CAD build for the part. Positions are in the model's coordinates, mm. A direction names the side the tool comes from. Give positions to 0.01 mm unless a question says otherwise; leave off trailing zeros. Order: outer loops, then holes, each group sorted by start corner. A loop starts at its lowest first (then second) coordinate and runs counter-clockwise, first axis right, second up.
```python
from build123d import *

# Parameters (mm, degrees)
SKETCH1_R           = 0.5
SKETCH1_R_2         = 1.375
BOSS_EXTRUDE1_DEPTH = 2
SKETCH4_R           = 4.6270037
SKETCH4_R_2         = 2.6270037
BOSS_EXTRUDE3_DEPTH = 6.5
CUT_EXTRUDE3_DEPTH  = 6.5
SKETCH6_R           = 15.875
SKETCH6_R_2         = 3.75
BOSS_EXTRUDE6_DEPTH = 2.54
SKETCH7_R           = 1.778
CUT_EXTRUDE4_DEPTH  = 2.54
CIRPATTERN1_COUNT   = 4
ESQUISSE1_R         = 15.875
ESQUISSE1_R_2       = 1.375
ESQUISSE1_R_3       = 1.778
BOSS_EXTRU_1_DEPTH  = 1.46
ESQUISSE2_R         = 4.625
BOSS_EXTRU_2_DEPTH  = 7.8


with BuildPart() as part:
    # Sketch1 → Boss-Extrude1 (new body)
    with BuildSketch(Plane(origin=(0, 0, 0), x_dir=(1, 0, 0), z_dir=(0, 1, 0))):
        with BuildLine():
            Line((-4, 4), (-2.467435953, 13.402193757))
            ThreePointArc((-2.467435953, 13.402193757), (0, 15.5), (2.467435953, 13.402193757))
            Line((2.467435953, 13.402193757), (4, 4))
            Line((4, 4), (12.448472752, 2.459445505))
            ThreePointArc((12.448472752, 2.459445505), (14.5, 0), (12.448472752, -2.459445505))
            Line((12.448472752, -2.459445505), (4, -4))
            Line((4, -4), (2.467435953, -13.402193757))
            ThreePointArc((2.467435953, -13.402193757), (0, -15.5), (-2.467435953, -13.402193757))
            Line((-2.467435953, -13.402193757), (-4, -4))
            Line((-4, -4), (-12.448472752, -2.459445505))
            ThreePointArc((-12.448472752, -2.459445505), (-14.5, 0), (-12.448472752, 2.459445505))
            Line((-12.448472752, 2.459445505), (-4, 4))
        make_face()
        with Locations((0, 12)):
            Circle(SKETCH1_R, mode=Mode.SUBTRACT)
        with Locations((0, 9.5)):
            Circle(SKETCH1_R, mode=Mode.SUBTRACT)
        with Locations((0, 7.5)):
            Circle(SKETCH1_R, mode=Mode.SUBTRACT)
        with Locations((12, 0)):
            Circle(SKETCH1_R, mode=Mode.SUBTRACT)
        with Locations((9.5, 0)):
            Circle(SKETCH1_R, mode=Mode.SUBTRACT)
        with Locations((7.5, 0)):
            Circle(SKETCH1_R, mode=Mode.SUBTRACT)
        with Locations((0, -12)):
            Circle(SKETCH1_R, mode=Mode.SUBTRACT)
        with Locations((0, -9.5)):
            Circle(SKETCH1_R, mode=Mode.SUBTRACT)
        with Locations((0, -7.5)):
            Circle(SKETCH1_R, mode=Mode.SUBTRACT)
        with Locations((-12, 0)):
            Circle(SKETCH1_R, mode=Mode.SUBTRACT)
        with Locations((-9.5, 0)):
            Circle(SKETCH1_R, mode=Mode.SUBTRACT)
        with Locations((-7.5, 0)):
            Circle(SKETCH1_R, mode=Mode.SUBTRACT)
        Circle(SKETCH1_R_2, mode=Mode.SUBTRACT)
    extrude(amount=BOSS_EXTRUDE1_DEPTH)

    # Sketch4 → Boss-Extrude3 (add)
    with BuildSketch(Plane.XZ):
        Circle(SKETCH4_R)
        Circle(SKETCH4_R_2, mode=Mode.SUBTRACT)
    extrude(amount=BOSS_EXTRUDE3_DEPTH)

    # Sketch5 → Cut-Extrude3 (cut)
    with BuildSketch(Plane.XZ.offset(6.5)):
        with BuildLine():
            Line((0.282820055, 2.611735296), (0, 3.101594))
            Line((0, 3.101594), (-0.282820055, 2.611735296))
            ThreePointArc((-0.282820055, 2.611735296), (0, 2.6270037), (0.282820055, 2.611735296))
        make_face()
        with BuildLine():
            ThreePointArc((-1.076048447, 2.396511669), (-0.811788788, 2.498428987), (-0.538092735, 2.571304075))
            Line((-0.538092735, 2.571304075), (-0.958445256, 2.949791185))
            Line((-0.958445256, 2.949791185), (-1.076048447, 2.396511669))
        make_face()
        with BuildLine():
            Line((0.958445256, 2.949791185), (0.538092735, 2.571304075))
            ThreePointArc((0.538092735, 2.571304075), (0.811788788, 2.498428987), (1.076048447, 2.396511669))
            Line((1.076048447, 2.396511669), (0.958445256, 2.949791185))
        make_face()
        with BuildLine():
            ThreePointArc((-1.76394572, 1.946700782), (-1.544114033, 2.125290638), (-1.306333259, 2.279175696))
            Line((-1.306333259, 2.279175696), (-1.823071212, 2.509242256))
            Line((-1.823071212, 2.509242256), (-1.76394572, 1.946700782))
        make_face()
        with BuildLine():
            Line((1.823071212, 2.509242256), (1.306333259, 2.279175696))
            ThreePointArc((1.306333259, 2.279175696), (1.544114033, 2.125290638), (1.76394572, 1.946700782))
            Line((1.76394572, 1.946700782), (1.823071212, 2.509242256))
        make_face()
        with BuildLine():
            ThreePointArc((-2.279175696, 1.306333259), (-2.125290638, 1.544114033), (-1.946700782, 1.76394572))
            Line((-1.946700782, 1.76394572), (-2.509242256, 1.823071212))
            Line((-2.509242256, 1.823071212), (-2.279175696, 1.306333259))
        make_face()
        with BuildLine():
            Line((2.509242256, 1.823071212), (1.946700782, 1.76394572))
            ThreePointArc((1.946700782, 1.76394572), (2.125290638, 1.544114033), (2.279175696, 1.306333259))
            Line((2.279175696, 1.306333259), (2.509242256, 1.823071212))
        make_face()
        with BuildLine():
            ThreePointArc((-2.571304075, 0.538092735), (-2.498428987, 0.811788788), (-2.396511669, 1.076048447))
            Line((-2.396511669, 1.076048447), (-2.949791185, 0.958445256))
            Line((-2.949791185, 0.958445256), (-2.571304075, 0.538092735))
        make_face()
        with BuildLine():
            Line((2.949791185, 0.958445256), (2.396511669, 1.076048447))
            ThreePointArc((2.396511669, 1.076048447), (2.498428987, 0.811788788), (2.571304075, 0.538092735))
            Line((2.571304075, 0.538092735), (2.949791185, 0.958445256))
        make_face()
        with BuildLine():
            ThreePointArc((-2.611735296, -0.282820055), (-2.6270037, 0), (-2.611735296, 0.282820055))
            Line((-2.611735296, 0.282820055), (-3.101594, 0))
            Line((-3.101594, 0), (-2.611735296, -0.282820055))
        make_face()
        with BuildLine():
            Line((3.101594, 0), (2.611735296, 0.282820055))
            ThreePointArc((2.611735296, 0.282820055), (2.6270037, 0), (2.611735296, -0.282820055))
            Line((2.611735296, -0.282820055), (3.101594, 0))
        make_face()
        with BuildLine():
            ThreePointArc((-2.396511669, -1.076048447), (-2.498428987, -0.811788788), (-2.571304075, -0.538092735))
            Line((-2.571304075, -0.538092735), (-2.949791185, -0.958445256))
            Line((-2.949791185, -0.958445256), (-2.396511669, -1.076048447))
        make_face()
        with BuildLine():
            Line((2.949791185, -0.958445256), (2.571304075, -0.538092735))
            ThreePointArc((2.571304075, -0.538092735), (2.498428987, -0.811788788), (2.396511669, -1.076048447))
            Line((2.396511669, -1.076048447), (2.949791185, -0.958445256))
        make_face()
        with BuildLine():
            ThreePointArc((-1.946700782, -1.76394572), (-2.125290638, -1.544114033), (-2.279175696, -1.306333259))
            Line((-2.279175696, -1.306333259), (-2.509242256, -1.823071212))
            Line((-2.509242256, -1.823071212), (-1.946700782, -1.76394572))
        make_face()
        with BuildLine():
            Line((2.509242256, -1.823071212), (2.279175696, -1.306333259))
            ThreePointArc((2.279175696, -1.306333259), (2.125290638, -1.544114033), (1.946700782, -1.76394572))
            Line((1.946700782, -1.76394572), (2.509242256, -1.823071212))
        make_face()
        with BuildLine():
            ThreePointArc((-1.306333259, -2.279175696), (-1.544114033, -2.125290638), (-1.76394572, -1.946700782))
            Line((-1.76394572, -1.946700782), (-1.823071212, -2.509242256))
            Line((-1.823071212, -2.509242256), (-1.306333259, -2.279175696))
        make_face()
        with BuildLine():
            Line((1.823071212, -2.509242256), (1.76394572, -1.946700782))
            ThreePointArc((1.76394572, -1.946700782), (1.544114033, -2.125290638), (1.306333259, -2.279175696))
            Line((1.306333259, -2.279175696), (1.823071212, -2.509242256))
        make_face()
        with BuildLine():
            ThreePointArc((-0.538092735, -2.571304075), (-0.811788788, -2.498428987), (-1.076048447, -2.396511669))
            Line((-1.076048447, -2.396511669), (-0.958445256, -2.949791185))
            Line((-0.958445256, -2.949791185), (-0.538092735, -2.571304075))
        make_face()
        with BuildLine():
            Line((0.958445256, -2.949791185), (1.076048447, -2.396511669))
            ThreePointArc((1.076048447, -2.396511669), (0.811788788, -2.498428987), (0.538092735, -2.571304075))
            Line((0.538092735, -2.571304075), (0.958445256, -2.949791185))
        make_face()
        with BuildLine():
            ThreePointArc((0.282820055, -2.611735296), (0, -2.6270037), (-0.282820055, -2.611735296))
            Line((-0.282820055, -2.611735296), (0, -3.101594))
            Line((0, -3.101594), (0.282820055, -2.611735296))
        make_face()
    extrude(amount=-CUT_EXTRUDE3_DEPTH, mode=Mode.SUBTRACT)

    # Sketch6 → Boss-Extrude6 (add)
    with BuildSketch(Plane(origin=(0, 2, 0), x_dir=(1, 0, 0), z_dir=(0, 1, 0))):
        Circle(SKETCH6_R)
        Circle(SKETCH6_R_2, mode=Mode.SUBTRACT)
    extrude(amount=-BOSS_EXTRUDE6_DEPTH)

    # Sketch7 → Cut-Extrude4 (cut)
    with BuildSketch(Plane(origin=(0, 2, 0), x_dir=(1, 0, 0), z_dir=(0, 1, 0))):
        with Locations((0, 9.779)):
            Circle(SKETCH7_R)
    cut_extrude4 = extrude(amount=-CUT_EXTRUDE4_DEPTH, mode=Mode.SUBTRACT)

    # CirPattern1: Cut-Extrude4 ×4 about axis
    cirpattern1_axis = Axis((0, 0, 0), (0, 1, 0))
    for i in range(1, CIRPATTERN1_COUNT):
        add(cut_extrude4.rotate(cirpattern1_axis, i * 360 / CIRPATTERN1_COUNT), mode=Mode.SUBTRACT)

    # Esquisse1 → Boss.-Extru.1 (add)
    with BuildSketch(Plane(origin=(0, 2, 0), x_dir=(1, 0, 0), z_dir=(0, 1, 0))):
        Circle(ESQUISSE1_R)
        Circle(ESQUISSE1_R_2, mode=Mode.SUBTRACT)
        with Locations((0, 9.779)):
            Circle(ESQUISSE1_R_3, mode=Mode.SUBTRACT)
        with Locations((9.779, 0)):
            Circle(ESQUISSE1_R_3, mode=Mode.SUBTRACT)
        with Locations((0, -9.779)):
            Circle(ESQUISSE1_R_3, mode=Mode.SUBTRACT)
        with Locations((-9.779, 0)):
            Circle(ESQUISSE1_R_3, mode=Mode.SUBTRACT)
    extrude(amount=BOSS_EXTRU_1_DEPTH)

    # Esquisse2 → Boss.-Extru.2 (add)
    with BuildSketch(Plane(origin=(0, 3.46, 0), x_dir=(1, 0, 0), z_dir=(0, 1, 0))):
        Circle(ESQUISSE2_R)
    extrude(amount=BOSS_EXTRU_2_DEPTH)


solid = part.part
```
Item 1: Tool access for faces 5 (the face through (3, -0.54, -4)), 6 (the face through (3, 3.46, -4)), 7 (the face through (0, 11.26, 0)): list every direction of +Z, -Z, +X, -X, +Y, -Y with a clear straight run to the whole face (end or side of a thin tool).
Item 2: Two-plate mould, pull along X, no slides. Class faces 1 (the face through (-1.003, 7.305, 4.515)), 2 (the face through (0, 3.46, 0)), 3 (the face through (0.73, 0, 1.34)), 4 (the face through (2, -6.5, -2)): released by +X, released by -X, zero draft, split by the parting line, or undercut.
Item 3: Drop flat-ended pins along their axis: pin 1 Ø1.9 at (x, z) = (0, 1) entering from -Y; pin 2 Ø2 at (y, z) = (3.5, -7) entering from +X; pin 3 Ø3 at (x, y) = (8.5, 3) entering from +Z. Give the stop position or say it passes through.
Item 4: Slice it at A-A (x = 11). Give the cut face in (y, z).
Item 5: Slice it at C-C (x = 7.5). Give the cut face in (y, z), and give its area (3 significant figures).
Item 6: Slice it at D-D (z = 6). Give the cut face in (x, y).
Item 7: Wall check: L1, parallel to X at y = 1.4, z = 0 (3 decimals); L2, parallel to X at y = 2.25, z = -1.5. Give the ranges that are in metal, low to high.
Item 8: Slice it at B-B (y = 8.75). Give the cut face in (x, z) (3 decimals), and give its area (3 significant figures).
A:
1. face 5: -Y
1. face 6: +Y
1. face 7: +Z, -Z, +X, -X, +Y
2. face 1: split by the parting line
2. face 2: undercut
2. face 3: undercut
2. face 4: zero draft
3. pin 1: stops at y = 0
3. pin 2: stops at x = 14.7
3. pin 3: stops at z = 14.25
4. outline: (-0.54, -11.45) - (3.46, -11.45) - (3.46, -1.29) - (-0.54, -1.29) - close; (-0.54, 1.29) - (3.46, 1.29) - (3.46, 11.45) - (-0.54, 11.45) - close
5. outline: (-0.54, -13.99) - (3.46, -13.99) - (3.46, 13.99) - (-0.54, 13.99) - close
5. area: 112 mm2
6. outline: (-14.7, -0.54) - (14.7, -0.54) - (14.7, 3.46) - (-14.7, 3.46) - close
7. L1: x = -15.875 to -11.557, -8.001 to -1.375, 1.375 to 8.001, 11.557 to 15.875
7. L2: x = -15.8 to -10.73, -8.82 to 8.82, 10.73 to 15.8
8. outline: circle Ø9.25 at (0, 0)
8. area: 67.2 mm2
